Input: dimensioned drawing with shaded views. Units: mm. Origin: part minimum x, y, z. A direction names the side the tool comes from. Coordinates: 2 decimals unless noted, no trailing zeros. Order: outer loops, then holes, each group sorted by start corner. A loop starts at its lowest first (then second) coordinate and runs counter-clockwise, first axis right, second up. Notation, with made-up numbers: (30, 15.25) -> (53, 15.25) arc R29 ccw to (53, 53.25) -> close; hole circle Ø10 at (69, 9). An arc over 180 degrees is marked (long way). Write item = value, one per line. Start each with the question number.
Item 1: Contact query for flat-ended pins moving along their axis: pin 1 (1.4 mm diameter, centred on x = 1.5, z = 2, fed in from -Y) (3 decimals); pin 2 (1.1 mm diameter, centred on x = 10.5, y = 1, fed in from +Z) (1 decimal); pin 3 (1.2 mm diameter, centred on x = 4, z = 2, fed in from +Y). Output: stop coordinate, or through.
Item 2: Section query B-B (x = 9.75). Output: boundary loops of the cut face in (y, z) (3 decimals).
Item 3: Mould query, pull axis Z, two halves, no side actions, for the marked faces 6, 7, 8 and 9. Classes: released by +Z, released by -Z, zero draft, split by the parting line, or undercut.
Item 4: Ray query, line 1 along X through (y, z) = (2.6, 2.45); line 2 along Z through (x, y) = (8.69, 2.05); line 3 along Z through (x, y) = (4, 1.25). Return the intervals inside material, ascending. Write a range as [from, to].
Item 5: Section query C-C (y = 1.1). Output: boundary loops of the cut face in (x, z) (1 decimal), then the cut area to 3 significant figures.
Item 6: Set-up query: the marked faces 1, 2, 3, 4 and 5. Return all of +Z, -Z, +X, -X, +Y, -Y with unobstructed straight access to the full face (end or side cutting, diameter ignored); none if empty.
Item 7: Section query D-D (x = 8). Output: boundary loops of the cut face in (y, z).
Item 8: Section query A-A (y = 0.6). Output: boundary loops of the cut face in (x, z) (1 decimal).
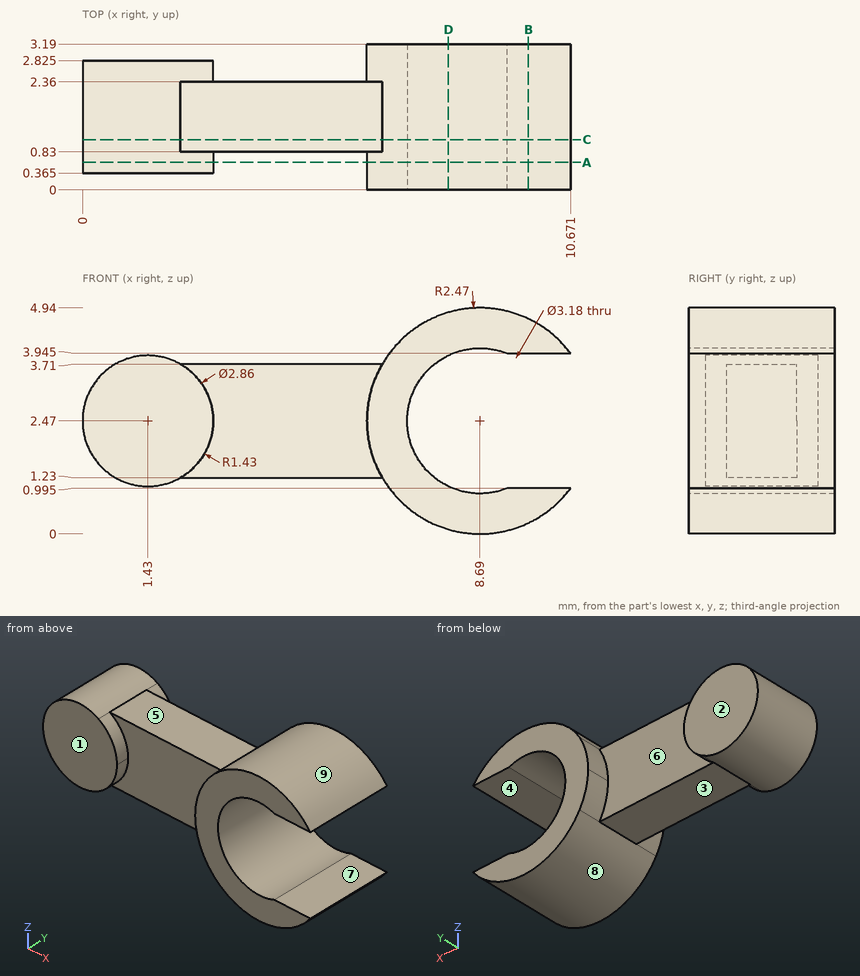
Computed:
q1.pin_1 = 0.365
q1.pin_2 = 4.6
q1.pin_3 = 2.36
q2.outline = (0, 0.239) -> (3.19, 0.239) -> (3.19, 0.995) -> (0, 0.995) -> close; (0, 3.945) -> (3.19, 3.945) -> (3.19, 4.701) -> (0, 4.701) -> close
q3.face_6 = zero draft
q3.face_7 = undercut
q3.face_8 = released by -Z
q3.face_9 = released by +Z
q4.line_1 = [0, 2.86], [6.22, 7.1]
q4.line_2 = [0, 0.88], [4.06, 4.94]
q4.line_3 = [1.23, 3.71]
q5.outline = (2.1, 1.2) -> (6.6, 1.2) arc R2.5 ccw to (10.7, 1) -> (9.3, 1) arc R1.6 cw (long way) to (9.3, 3.9) -> (10.7, 3.9) arc R2.5 ccw to (6.6, 3.7) -> (2.1, 3.7) arc R1.4 ccw (long way) to start
q5.area = 23.8 mm^2
q6.face_1 = +Z, -Z, -X, -Y
q6.face_2 = +Z, -Z, -X, +Y
q6.face_3 = -Z, +Y, -Y
q6.face_4 = +X, +Y, -Y
q6.face_5 = +Z, +Y, -Y
q7.outline = (0, 0.1) -> (3.19, 0.1) -> (3.19, 1.04) -> (0, 1.04) -> close; (0, 3.9) -> (3.19, 3.9) -> (3.19, 4.84) -> (0, 4.84) -> close
q8.outline = circle Ø2.9 at (1.4, 2.5); (6.2, 2.5) arc R2.5 ccw to (6.6, 1.2) arc R2.5 ccw to (10.7, 1) -> (9.3, 1) arc R1.6 cw (long way) to (9.3, 3.9) -> (10.7, 3.9) arc R2.5 ccw to (6.6, 3.7) arc R2.5 ccw to start
